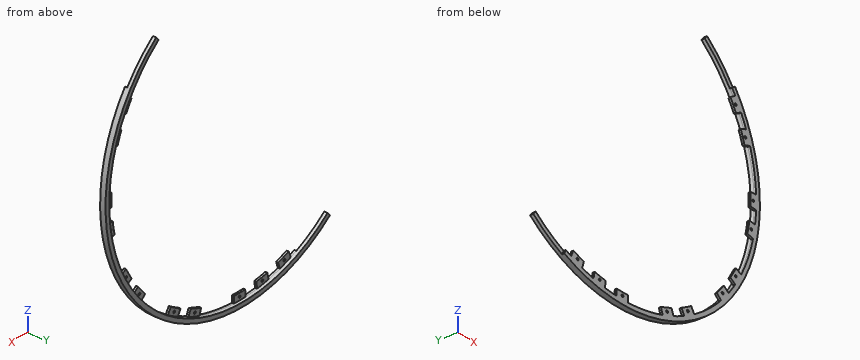
```python
from build123d import *

# Parameters (mm, degrees)
F_3_8_CLEARANCE_HOLE1_D = 10.31748
CUT_EXTRUDE1_DEPTH      = 1044.898713202
CIRPATTERN1_COUNT       = 36
CUT_EXTRUDE_THIN1_START = -10.16
CUT_EXTRUDE_THIN1_DEPTH = 1055.247002027
CIRPATTERN3_COUNT       = 2
CUT_EXTRUDE3_DEPTH      = 1045.087002027
CUT_EXTRUDE4_DEPTH      = 1045.087002027


with BuildPart() as part:
    # Sketch1 → Revolve1 (revolve)
    with BuildSketch(Plane.XY, mode=Mode.PRIVATE) as revolve1_sk:
        Polygon((687.262499996, 0), (687.262499996, -9.525), (738.062499996, -9.525), (738.062499996, 0), (738.062499996, 15.875), (718.17500002, 15.875), (718.17500002, 0), align=None)
    revolve(revolve1_sk.sketch.rotate(Axis((0, 57.350368034, 0), (0, -1, 0)), 90), axis=Axis((0, 57.350368034, 0), (0, -1, 0)))

    # 3/8 Clearance Hole1 (through all)
    with Locations(Plane(origin=(0, 0, 0), x_dir=(1, 0, 0), z_dir=(0, 1, 0))):
        with Locations((702.500000128, 0)):
            f_3_8_clearance_hole1 = Hole(F_3_8_CLEARANCE_HOLE1_D / 2)

    # Sketch16 → Cut-Extrude1 (cut, through all)
    with BuildSketch(Plane(origin=(0, 0, 0), x_dir=(1, 0, 0), z_dir=(0, 1, 0))):
        with BuildLine():
            Line((712.030913337, -93.7406481), (681.382874036, -89.70575718))
            Line((681.382874036, -89.70575718), (0, 0))
            Line((0, 0), (686.608378381, -29.977969209))
            Line((686.608378381, -29.977969209), (717.491456555, -31.326353522))
            ThreePointArc((717.491456555, -31.326353522), (715.442127322, -62.59307555), (712.030913337, -93.7406481))
        make_face()
    cut_extrude1 = extrude(amount=-CUT_EXTRUDE1_DEPTH, mode=Mode.SUBTRACT)

    # CirPattern1: 3/8 Clearance Hole1, Cut-Extrude1 ×36 about axis
    cirpattern1_axis = Axis((0, 0, 0), (0, 1, 0))
    add([f_3_8_clearance_hole1.rotate(cirpattern1_axis, i * 360 / CIRPATTERN1_COUNT) for i in range(1, CIRPATTERN1_COUNT)], mode=Mode.SUBTRACT)
    add([cut_extrude1.rotate(cirpattern1_axis, i * 360 / CIRPATTERN1_COUNT) for i in range(1, CIRPATTERN1_COUNT)], mode=Mode.SUBTRACT)

    # Sketch18 → Cut-Extrude-Thin1 (cut)
    with BuildSketch(Plane.XZ.offset(9.525).offset(CUT_EXTRUDE_THIN1_START)):
        with BuildLine():
            ThreePointArc((314.248373982, 673.907812764), (477.960796886, 569.611496808), (609.100981349, 426.497098671))
            Line((609.100981349, 426.497098671), (557.084826536, 390.074994963))
            ThreePointArc((557.084826536, 390.074994963), (437.14378367, 520.967674669), (287.412114362, 616.357268287))
            Line((287.412114362, 616.357268287), (314.248373982, 673.907812764))
        make_face()
    cut_extrude_thin1 = extrude(amount=CUT_EXTRUDE_THIN1_DEPTH, mode=Mode.SUBTRACT)

    # CirPattern3: Cut-Extrude-Thin1 ×2 about axis
    cirpattern3_axis = Axis((0, 0, 0), (0, 1, 0))
    for i in range(1, CIRPATTERN3_COUNT):
        add(cut_extrude_thin1.rotate(cirpattern3_axis, i * 360 / CIRPATTERN3_COUNT), mode=Mode.SUBTRACT)

    # Sketch41 → Cut-Extrude3 (cut, through all)
    with BuildSketch(Plane.XZ.offset(9.525)):
        with BuildLine():
            Line((693.703780314, 185.877367722), (663.844598186, 177.876623984))
            ThreePointArc((663.844598186, 177.876623984), (676.821438351, 119.341880703), (684.647258693, 59.89887365))
            Line((684.647258693, 59.89887365), (715.442127322, 62.59307555))
            ThreePointArc((715.442127322, 62.59307555), (707.264308039, 124.709779999), (693.703780314, 185.877367722))
        make_face()
        with BuildLine():
            Line((693.703780314, -185.877367722), (663.844598186, -177.876623984))
            ThreePointArc((663.844598186, -177.876623984), (645.815499789, -235.057618751), (622.871355485, -290.449683108))
            Line((622.871355485, -290.449683108), (650.887594973, -303.513870134))
            ThreePointArc((650.887594973, -303.513870134), (674.863747952, -245.63031644), (693.703780314, -185.877367722))
        make_face()
        with BuildLine():
            Line((507.826412593, -507.826412593), (485.967974202, -485.967974202))
            ThreePointArc((485.967974202, -485.967974202), (441.7638196, -526.473619086), (394.197575585, -562.972481835))
            Line((394.197575585, -562.972481835), (411.928257188, -588.294519424))
            ThreePointArc((411.928257188, -588.294519424), (461.633991599, -550.153967952), (507.826412593, -507.826412593))
        make_face()
        with BuildLine():
            Line((185.877367722, -693.703780314), (177.876623984, -663.844598186))
            ThreePointArc((177.876623984, -663.844598186), (119.341880703, -676.821438351), (59.89887365, -684.647258693))
            Line((59.89887365, -684.647258693), (62.593075549, -715.442127322))
            ThreePointArc((62.593075549, -715.442127322), (124.709779999, -707.264308039), (185.877367722, -693.703780314))
        make_face()
        with BuildLine():
            Line((-693.703780315, -185.877367721), (-663.844598186, -177.876623984))
            ThreePointArc((-663.844598186, -177.876623984), (-676.821438351, -119.341880703), (-684.647258693, -59.89887365))
            Line((-684.647258693, -59.89887365), (-715.442127322, -62.593075549))
            ThreePointArc((-715.442127322, -62.593075549), (-707.264308039, -124.709779999), (-693.703780315, -185.877367721))
        make_face()
        with BuildLine():
            Line((-693.703780314, 185.877367722), (-663.844598186, 177.876623984))
            ThreePointArc((-663.844598186, 177.876623984), (-645.815499789, 235.057618751), (-622.871355485, 290.449683108))
            Line((-622.871355485, 290.449683108), (-650.887594973, 303.513870134))
            ThreePointArc((-650.887594973, 303.513870134), (-674.863747952, 245.63031644), (-693.703780314, 185.877367722))
        make_face()
        with BuildLine():
            Line((-507.826412593, 507.826412593), (-485.967974202, 485.967974203))
            ThreePointArc((-485.967974202, 485.967974203), (-441.763819599, 526.473619086), (-394.197575585, 562.972481835))
            Line((-394.197575585, 562.972481835), (-411.928257188, 588.294519424))
            ThreePointArc((-411.928257188, 588.294519424), (-461.633991599, 550.153967952), (-507.826412593, 507.826412593))
        make_face()
        with BuildLine():
            Line((-185.877367721, 693.703780315), (-177.876623983, 663.844598186))
            ThreePointArc((-177.876623983, 663.844598186), (-119.341880703, 676.821438351), (-59.898873649, 684.647258693))
            Line((-59.898873649, 684.647258693), (-62.593075549, 715.442127322))
            ThreePointArc((-62.593075549, 715.442127322), (-124.709779999, 707.264308039), (-185.877367721, 693.703780315))
        make_face()
    extrude(amount=-CUT_EXTRUDE3_DEPTH, mode=Mode.SUBTRACT)

    # Sketch42 → Cut-Extrude4 (cut, through all)
    with BuildSketch(Plane(origin=(0, 15.875, 0), x_dir=(1, 0, 0), z_dir=(0, 1, 0))):
        with BuildLine():
            ThreePointArc((-466.098832167, 572.265788383), (-572.265788383, -466.098832167), (466.098832167, -572.265788383))
            Line((466.098832167, -572.265788383), (453.539542793, -556.845771985))
            ThreePointArc((453.539542793, -556.845771984), (240.689237761, -676.64172313), (0, -718.17500002))
            ThreePointArc((0, -718.17500002), (-31.326353522, -717.491456555), (-62.593075549, -715.442127322))
            ThreePointArc((-62.593075549, -715.442127322), (-124.709779999, -707.264308039), (-185.877367721, -693.703780315))
            ThreePointArc((-185.877367721, -693.703780315), (-303.513870134, -650.887594973), (-411.928257188, -588.294519424))
            ThreePointArc((-411.928257188, -588.294519424), (-461.633991599, -550.153967952), (-507.826412593, -507.826412593))
            ThreePointArc((-507.826412593, -507.826412593), (-588.294519423, -411.928257188), (-650.887594973, -303.513870134))
            ThreePointArc((-650.887594973, -303.513870134), (-674.863747952, -245.63031644), (-693.703780314, -185.877367722))
            ThreePointArc((-693.703780314, -185.877367722), (-715.442127322, -62.59307555), (-715.442127322, 62.593075549))
            ThreePointArc((-715.442127322, 62.593075549), (-707.264308039, 124.709779999), (-693.703780315, 185.877367721))
            ThreePointArc((-693.703780315, 185.877367721), (-602.864993049, 390.293646899), (-453.539542793, 556.845771984))
            Line((-453.539542793, 556.845771985), (-466.098832167, 572.265788383))
        make_face()
    extrude(amount=-CUT_EXTRUDE4_DEPTH, mode=Mode.SUBTRACT)


with BuildPart() as cut_extrude4_kept_piece:
    # of the separate pieces the step leaves, the one the design keeps (cut_extrude4_pieces_kept)
    add(part.part.solids().sort_by_distance((-311.918690804, -9.525, -668.911791066))[0])


solid = cut_extrude4_kept_piece.part
```
Verification items for the finished model (mm, model axes). Coordinates: 2 decimals unless noted, no trailing zeros. Order: outer loops, then holes, each group sorted by start corner. A loop starts at its lowest first (then second) coordinate and runs counter-clockwise, first axis right, second up. Notation, with made-up numbers: (75, 64) - (108, 64) arc R33 ccw to (108, 99) - close; hole circle Ø2 at (59, 24.25). An arc over 180 degrees is marked (long way). Return JSON: item names as keys, results as strings.
(1) Go/stop test with flat-tipped pins: pin 1 (9.5 mm diameter, centred on x = 702.5, z = 0, fed in from +Y); pin 2 (9.5 mm diameter, centred on x = 709.5, z = 0, fed in from +Y); pin 3 (8 mm diameter, centred on x = -227.5, y = -7, fed in from -Z); pin 4 (12 mm diameter, centred on x = 468.5, y = -2.5, fed in from -Z). Record where each tip stops, or that it passes through.
Filled sheet:
{"pin 1": "passes through", "pin 2": "stops at y = 0", "pin 3": "stops at z = -703.41", "pin 4": "stops at z = -575.18"}
(2) Thickness scan on line 1 along Z through (x, y) = (584, -6.5); line 2 along Z through (x, y) = (19, -5.75); line 3 along Z through (x, y) = (600.5, 1.75). Record the ranges inside material, lowest first.
Filled sheet:
{"line 1": "z = -451.31 to -417.99, -372.05 to -362.32, 362.32 to 372.05", "line 2": "z = -737.82 to -687", "line 3": "z = -429.11 to -393.92, 393.92 to 429.11"}
(3) Section check B-B, the plane z = 460. Record the cut outline in (x, y) (3 decimals), and give its area (3 significant figures).
Filled sheet:
{"outline": "(551.521, 0.635) - (577.18, 0.635) - (577.18, 15.875) - (551.521, 15.875) - close", "area": "391 mm^2"}
(4) Section check C-C, the plane z = -248.5. Record the cut outline in (x, y) (1 decimal).
Filled sheet:
{"outline": "(673.8, -9.5) - (695, -9.5) - (695, 15.9) - (673.8, 15.9) - close"}
